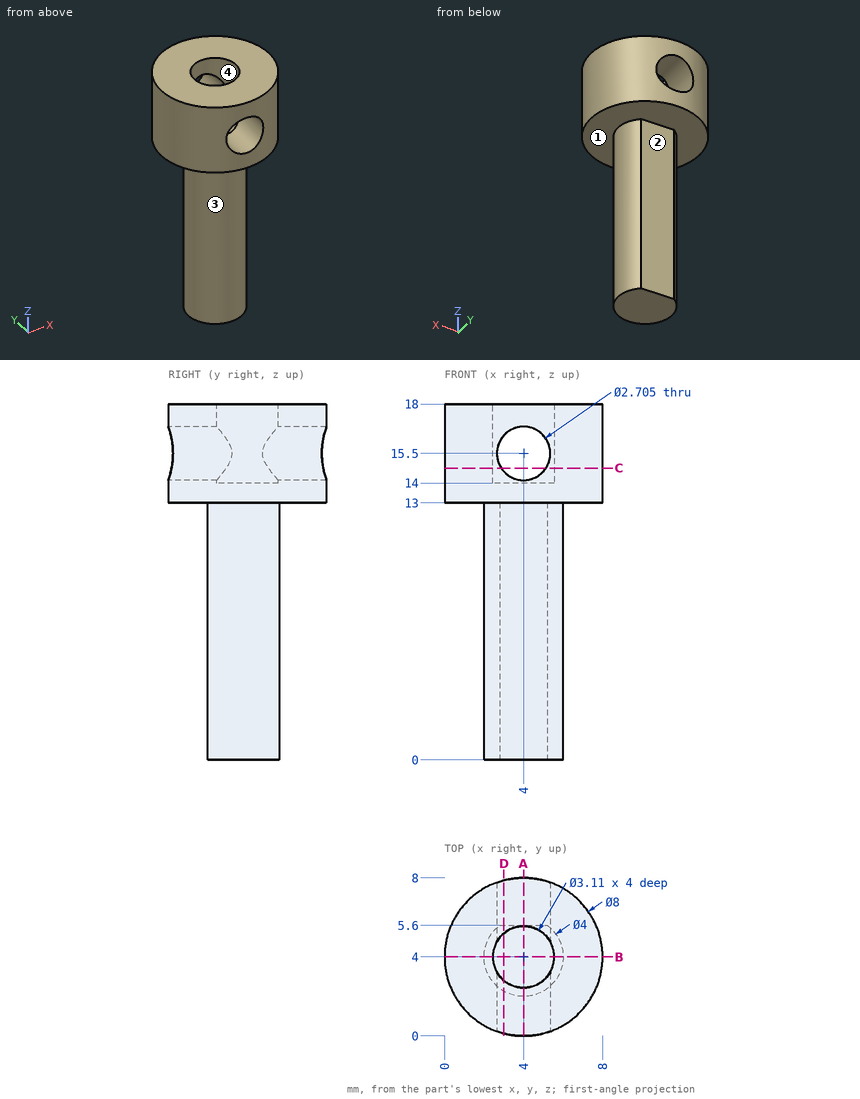
Part print with two shaded views. Sizes in mm from the minimum x, y, z corner. Round coordinates to 2 decimals unless told otherwise and drop trailing zeros. Order: outer loops, then holes, each group sorted by start corner. A loop starts at its lowest first (then second) coordinate and runs counter-clockwise, first axis right, second up. Notation, with made-up numbers: (38, -6) - (49, -6) arc R34 cw to (49, 31) - close; hole circle Ø11 at (53, 36.5). An arc over 180 degrees is marked (long way). Return JSON: item names as keys, results as strings.
(1) Cut at D-D (x = 3). Give the cut face in (y, z).
Answer key:
{"outline": "(0.13, 13) - (2.27, 13) - (2.27, 0) - (5.6, 0) - (5.6, 13) - (7.87, 13) - (7.87, 14.59) - (5.19, 14.59) - (5.19, 14) - (2.81, 14) - (2.81, 14.59) - (0.13, 14.59) - close; (0.13, 16.41) - (2.81, 16.41) - (2.81, 18) - (0.13, 18) - close; (5.19, 16.41) - (7.87, 16.41) - (7.87, 18) - (5.19, 18) - close"}
(2) Cut at B-B (y = 4). Give the cut face in (x, z) (3 decimals).
Answer key:
{"outline": "(0, 13) - (2, 13) - (2, 0) - (6, 0) - (6, 13) - (8, 13) - (8, 18) - (5.555, 18) - (5.555, 14) - (2.445, 14) - (2.445, 18) - (0, 18) - close"}
(3) Cut at C-C (z = 14.75). Give the cut face in (x, y) (1 decimal).
Answer key:
{"outline": "(2.9, 0.2) - (2.9, 2.9) arc R1.6 cw to (2.9, 5.1) - (2.9, 7.8) arc R4 ccw to start; (5.1, 0.2) arc R4 ccw to (5.1, 7.8) - (5.1, 5.1) arc R1.6 cw to (5.1, 2.9) - close"}
(4) Pin check, flat tips, straight feed: pin 1 Ø1.9 at (x, y) = (4, 4) entering from +Z; pin 2 Ø2.5 at (x, z) = (4, 15.5) entering from -Y; pin 3 Ø0.7 at (x, z) = (4, 7) entering from +Y; pin 4 Ø1.5 at (x, y) = (5, 6.5) entering from -Z. Stop position of each tip, or through.
Answer key:
{"pin 1": "stops at z = 14", "pin 2": "passes through", "pin 3": "stops at y = 5.6", "pin 4": "stops at z = 13"}
(5) Wall check: probe 1 along Z at (x, y) = (4, 1.25); probe 2 along Z at (x, y) = (2, 6.75); probe 3 along X at (y, z) = (1.85, 15.5). Give the ranges that are in metal, low to high. Write a range as from..to.
Answer key:
{"probe 1": "z = 13..14.15, 16.85..18", "probe 2": "z = 13..18", "probe 3": "x = 0.63..2.65, 5.35..7.37"}
(6) Cut at A-A (x = 4). State how many separate pieces and enclosed holes the cut face has, then the cut area to 3 significant figures.
Answer key:
{"separate pieces": "3", "enclosed holes": "0", "area": "61.1 mm^2"}
(7) Pull direction Y, two halves, no side cores. Call the marked faces 1, 2, 3 and 4: +Y half, -Y half, draft (parallel to the pull), parting line (faces both ways), or undercut.
Answer key:
{"face 1": "draft", "face 2": "+Y half", "face 3": "parting line", "face 4": "undercut"}
